Part model, mm, in its own coordinate system. Face numbers are marked on the shaded views. A direction names the side the tool comes from. Coordinates: 2 decimals unless noted, no trailing zeros. Loops run counter-clockwise (first coordinate to the right, second up) from the corner with the lowest first, then second, coordinate; pieces in that order, holes last. Notation, with made-up numbers: (74, 4.25) -> (121, 4.25) arc R24 ccw to (121, 22.25) -> close; hole circle Ø6 at (43, -4). An arc over 180 degrees is marked (long way). One line per question, with ' | ' between items. Start each with the question number.
1) Cut at C-C (y = -99). List the corners of the cut face in (x, z).
2) 3-axis set-ups, long thin cutter, end or side, ignore diameter. For the marked faces 4 and 5: which of +Z, -Z, +X, -X, +Y, -Y reach the whole face in a straight line?
3) Probe L1, parallel to Y at x = 103, z = 76.5; L2, parallel to X at y = -19.5, z = 8.5; L3, parallel to Z at x = 136, y = -42.5. List the from-to ranges inside material, lowest first. Write a range as from..to.
4) Cut at A-A (z = 82.5). List the corners of the cut face in (x, y), plus the area to 4 significant figures.
5) Cut at B-B (x = 135). List the corners of the cut face in (y, z), plus the area to 4 significant figures.
6) Drop flat-ended pins along their axis: pin 1 (1.2 mm diameter, centred on x = 153.5, y = -22.5, fed in from -Z); pin 2 (8 mm diameter, centred on x = -20.5, y = -89, fed in from +Z); pin 3 (6 mm diameter, centred on x = 95, z = 98, fed in from -Y). Give the stop position or say it passes through.
7) Two-plate mould, pull along Y, no slides. Class the marked faces 1, 2 and 3: released by +Y, released by -Y, zero draft, split by the parting line, or undercut.
from build123d import *

# Parameters (mm, degrees)
F0_W     = 310
F0_H     = 230
F1_DEPTH = 5
F2_W     = 310
F2_H     = 230
F2_W_2   = 305
F2_H_2   = 225
F3_DEPTH = 150
F4_W     = 210
F4_H     = 17
F5_DEPTH = 310.001
F6_W     = 290
F6_H     = 17
F7_DEPTH = 230.001


with BuildPart() as f1:
    # F0 (on Top) → F1 (new body)
    with BuildSketch(Plane.XY):
        Rectangle(F0_W, F0_H)
    extrude(amount=F1_DEPTH)

    # F2 (on face) → F3 (join)
    with BuildSketch(Plane(origin=(0, 0, 0), x_dir=(1, 0, 0), z_dir=(0, 0, -1))):
        Rectangle(F2_W, F2_H)
        Rectangle(F2_W_2, F2_H_2, mode=Mode.SUBTRACT)
    extrude(amount=-F3_DEPTH)

    # F4 (on face) → F5 (cut, through all)
    with BuildSketch(Plane(origin=(-155, 0, 0), x_dir=(0, -1, 0), z_dir=(-1, 0, 0))):
        with Locations((0, 102.5)):
            Rectangle(F4_W, F4_H)
        with Locations((0, 47.5)):
            Rectangle(F4_W, F4_H)
    extrude(amount=-F5_DEPTH, mode=Mode.SUBTRACT)

    # F6 (on face) → F7 (cut, through all)
    with BuildSketch(Plane.XZ.offset(115)):
        with Locations((0, 102.5)):
            Rectangle(F6_W, F6_H)
        with Locations((0, 47.5)):
            Rectangle(F6_W, F6_H)
    extrude(amount=-F7_DEPTH, mode=Mode.SUBTRACT)


solid = f1.part
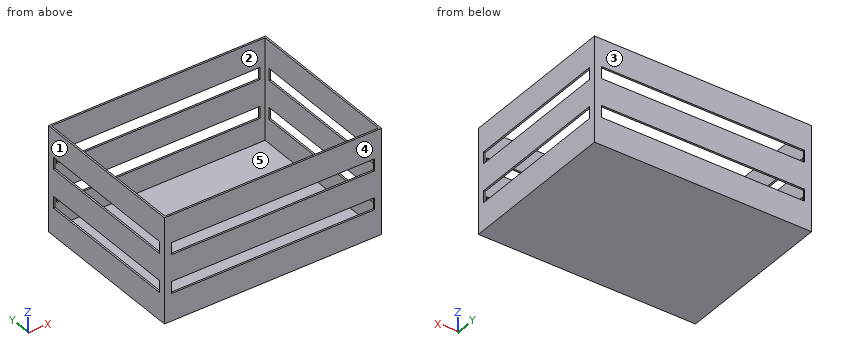
Reported:
1) outline: (-155, 0) -> (155, 0) -> (155, 39) -> (152.5, 39) -> (152.5, 5) -> (-152.5, 5) -> (-152.5, 39) -> (-155, 39) -> close; (-155, 56) -> (-152.5, 56) -> (-152.5, 94) -> (-155, 94) -> close; (-155, 111) -> (-152.5, 111) -> (-152.5, 150) -> (-155, 150) -> close; (152.5, 56) -> (155, 56) -> (155, 94) -> (152.5, 94) -> close; (152.5, 111) -> (155, 111) -> (155, 150) -> (152.5, 150) -> close
2) face 4: +Z, -Z, +X, -X, -Y | face 5: +Z
3) L1: y = -115..-112.5, 112.5..115 | L2: x = -155..-152.5, 152.5..155 | L3: z = 0..5
4) outline: (-155, -115) -> (155, -115) -> (155, 115) -> (-155, 115) -> close; hole (-152.5, -112.5) -> (152.5, -112.5) -> (152.5, 112.5) -> (-152.5, 112.5) -> close | area: 2,675 mm²
5) outline: (-115, 0) -> (115, 0) -> (115, 39) -> (112.5, 39) -> (112.5, 5) -> (-112.5, 5) -> (-112.5, 39) -> (-115, 39) -> close; (-115, 56) -> (-112.5, 56) -> (-112.5, 94) -> (-115, 94) -> close; (-115, 111) -> (-112.5, 111) -> (-112.5, 150) -> (-115, 150) -> close; (112.5, 56) -> (115, 56) -> (115, 94) -> (112.5, 94) -> close; (112.5, 111) -> (115, 111) -> (115, 150) -> (112.5, 150) -> close | area: 1,705 mm²
6) pin 1: stops at z = 0 | pin 2: stops at z = 5 | pin 3: passes through
7) face 1: zero draft | face 2: undercut | face 3: released by +Y
